```python
from build123d import *

# Parameters (mm, degrees)
SKETCH1_R           = 1.5
BOSS_EXTRUDE1_DEPTH = 25
SKETCH2_R           = 1.5
BOSS_EXTRUDE2_DEPTH = 2
SKETCH3_W           = 3
SKETCH3_H           = 17
CUT_EXTRUDE1_DEPTH  = 2
LPATTERN1_COUNT     = 7
LPATTERN1_PITCH     = 15


with BuildPart() as part:
    # Sketch1 → Boss-Extrude1 (new body)
    with BuildSketch(Plane.XY):
        with BuildLine():
            Line((-50.08587988, 100), (-70, 100))
            Line((-70, 100), (-70, -25.358547654))
            Line((-70, -25.358547654), (70, -25.358547654))
            Line((70, -25.358547654), (70, 30.840200363))
            ThreePointArc((70, 30.840200363), (67.647784394, 33.77119445), (66.543566366, 37.363456571))
            ThreePointArc((66.543566366, 37.363456571), (64.816659948, 40.011839547), (61.659897736, 40.187880739))
            ThreePointArc((61.659897736, 40.187880739), (57.09391383, 39.362702083), (52.647005809, 40.687140793))
            Line((52.647005809, 40.687140793), (21.252340591, 58.812859207))
            ThreePointArc((21.252340591, 58.812859207), (17.881889013, 62.001775167), (16.313522739, 66.368622551))
            ThreePointArc((16.313522739, 66.368622551), (14.584936491, 69.013139721), (11.430424316, 69.187880739))
            ThreePointArc((11.430424316, 69.187880739), (6.864440411, 68.362702083), (2.41753239, 69.687140793))
            Line((2.41753239, 69.687140793), (-28.977132828, 87.812859207))
            ThreePointArc((-28.977132828, 87.812859207), (-32.347584407, 91.001775167), (-33.915950681, 95.368622551))
            ThreePointArc((-33.915950681, 95.368622551), (-35.644536929, 98.013139721), (-38.799049103, 98.187880739))
            ThreePointArc((-38.799049103, 98.187880739), (-43.365033009, 97.362702083), (-47.81194103, 98.687140793))
            Line((-47.81194103, 98.687140793), (-50.08587988, 100))
        make_face()
        with BuildLine():
            Line((-50.621778265, 98), (68, 29.513684387))
            Line((68, 29.513684387), (68, -15.130655325))
            Line((68, -15.130655325), (51.241660417, -23.358547654))
            Line((51.241660417, -23.358547654), (-61.699771159, -23.358547654))
            Line((-61.699771159, -23.358547654), (-61.699771159, -19.718666382))
            ThreePointArc((-61.699771159, -19.718666382), (-63.017790644, -16.536685867), (-66.199771159, -15.218666382))
            Line((-66.199771159, -15.218666382), (-68, -15.218666382))
            Line((-68, -15.218666382), (-68, 98))
            Line((-68, 98), (-50.621778265, 98))
        make_face(mode=Mode.SUBTRACT)
        with Locations((63.06440991, 36.982050808)):
            Circle(SKETCH1_R, mode=Mode.SUBTRACT)
        with Locations((-37.394536929, 94.982050808)):
            Circle(SKETCH1_R, mode=Mode.SUBTRACT)
        with Locations((12.834936491, 65.982050808)):
            Circle(SKETCH1_R, mode=Mode.SUBTRACT)
        with Locations((65.552729719, -21.188668784)):
            Circle(SKETCH1_R, mode=Mode.SUBTRACT)
        with Locations((-66.199771159, -19.718666382)):
            Circle(SKETCH1_R, mode=Mode.SUBTRACT)
    extrude(amount=BOSS_EXTRUDE1_DEPTH)

    # Sketch2 → Boss-Extrude2 (add)
    with BuildSketch(Plane.XY.offset(25)):
        with BuildLine():
            Line((70, -25.358547654), (70, 30.840200363))
            ThreePointArc((70, 30.840200363), (67.647784394, 33.77119445), (66.543566366, 37.363456571))
            ThreePointArc((66.543566366, 37.363456571), (64.816659948, 40.011839547), (61.659897736, 40.187880739))
            ThreePointArc((61.659897736, 40.187880739), (57.09391383, 39.362702083), (52.647005809, 40.687140793))
            Line((52.647005809, 40.687140793), (21.252340591, 58.812859207))
            ThreePointArc((21.252340591, 58.812859207), (17.881889013, 62.001775167), (16.313522739, 66.368622551))
            ThreePointArc((16.313522739, 66.368622551), (14.584936491, 69.013139721), (11.430424316, 69.187880739))
            ThreePointArc((11.430424316, 69.187880739), (6.864440411, 68.362702083), (2.41753239, 69.687140793))
            Line((2.41753239, 69.687140793), (-28.977132828, 87.812859207))
            ThreePointArc((-28.977132828, 87.812859207), (-32.347584407, 91.001775167), (-33.915950681, 95.368622551))
            ThreePointArc((-33.915950681, 95.368622551), (-35.644536929, 98.013139721), (-38.799049103, 98.187880739))
            ThreePointArc((-38.799049103, 98.187880739), (-43.365033009, 97.362702083), (-47.81194103, 98.687140793))
            Line((-47.81194103, 98.687140793), (-50.08587988, 100))
            Line((-50.08587988, 100), (-70, 100))
            Line((-70, 100), (-70, -25.358547654))
            Line((-70, -25.358547654), (70, -25.358547654))
        make_face()
        with Locations((-37.394536929, 94.982050808)):
            Circle(SKETCH2_R, mode=Mode.SUBTRACT)
        with Locations((12.834936491, 65.982050808)):
            Circle(SKETCH2_R, mode=Mode.SUBTRACT)
        with Locations((63.06440991, 36.982050808)):
            Circle(SKETCH2_R, mode=Mode.SUBTRACT)
        with Locations((65.552729719, -21.188668784)):
            Circle(SKETCH2_R, mode=Mode.SUBTRACT)
        with Locations((-66.199771159, -19.718666382)):
            Circle(SKETCH2_R, mode=Mode.SUBTRACT)
    extrude(amount=BOSS_EXTRUDE2_DEPTH)

    # Sketch3 → Cut-Extrude1 (cut)
    with BuildSketch(Plane(origin=(0, -25.358547654, 0), x_dir=(-1, 0, 0), z_dir=(0, -1, 0))):
        with Locations((48.5, -13.5)):
            Rectangle(SKETCH3_W, SKETCH3_H)
    cut_extrude1 = extrude(amount=-CUT_EXTRUDE1_DEPTH, mode=Mode.SUBTRACT)

    # LPattern1: Cut-Extrude1 ×7
    with Locations(*[(i * LPATTERN1_PITCH, 0, 0) for i in range(1, LPATTERN1_COUNT)]):
        add(cut_extrude1, mode=Mode.SUBTRACT)


solid = part.part
```
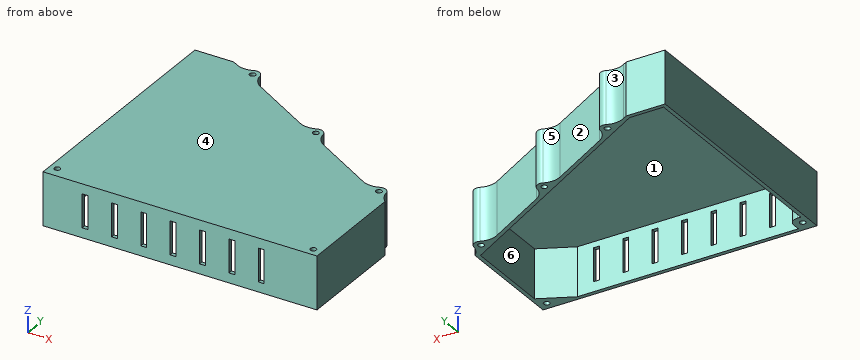
Work out the finished part from the listing and answer in its coordinate system (mm). Face numbers are marked on the shaded views. A direction names the side the tool comes from. Coordinates: 2 decimals unless noted, no trailing zeros. Loops run counter-clockwise (first coordinate to the right, second up) from the corner with the lowest first, then second, coordinate; pieces in that order, holes last. Notation, with made-up numbers: (-9, -20) -> (27, -20) arc R15 ccw to (27, -13) -> close; hole circle Ø8 at (51.5, 33). An arc over 180 degrees is marked (long way). Answer as CSV lines item,"result".
Q1. For a pull along X with two mould halves and no side action, classify the marked faces 1, 2, 3 and 4 as +X half, -X half, draft (parallel to the pull), parting line (faces both ways), or undercut.
Findings:
face 1,"undercut"
face 2,"+X half"
face 3,"undercut"
face 4,"draft"
Q2. A tool of negligible diameter and unlimited length cuts with its end or side. For the marked faces 5 and 6, from which of +Z, -Z, +X, -X, +Y, -Y can it reach the whole face along a straight path? Write none if from no direction.
Findings:
face 5,"+Z, -Z, +Y"
face 6,"-Z"
Q3. The part is cut by section C-C on z = 13. State how many separate pieces and enclosed holes the cut face has, and give its area (3 significant figures).
Findings:
separate pieces,"7"
enclosed holes,"5"
area,"1,130 mm²"
Q4. The part is cut by section B-B on y = 49. Write down the section's boundary in (x, z), and give its area (3 significant figures).
Findings:
outline,"(-70, 0) -> (-68, 0) -> (-68, 25) -> (34.25, 25) -> (34.25, 0) -> (38.25, 0) -> (38.25, 27) -> (-70, 27) -> close"
area,"366 mm²"
Q5. The part is cut by section A-A on x = -57.5. Write down the section's boundary in (y, z), and give its area (3 significant figures).
Findings:
outline,"(-25.36, 0) -> (-23.36, 0) -> (-23.36, 25) -> (98, 25) -> (98, 0) -> (100, 0) -> (100, 27) -> (-25.36, 27) -> close"
area,"351 mm²"
Q6. Find the intervals of material crossed by probe 1 along X at (y, z) = (-12.5, 20.25); probe 2 along X at (y, z) = (-19, 2); probe 3 along X at (y, z) = (-16, 18), in increasing order.
Findings:
probe 1,"x = -70 to -68, 68 to 70"
probe 2,"x = -70 to -67.52, -64.88 to -61.76, 60.12 to 70"
probe 3,"x = -70 to -63.67, 66.23 to 70"
Q7. Each of these flat-tipped pins is pushed along its axis until it touches: pin 1 (6 mm diameter, centred on x = 54, z = 16.5, fed in from +Y); pin 2 (1 mm diameter, centred on y = 35, z = 4, fed in from +X); pin 3 (12 mm diameter, centred on x = -41.5, z = 10, fed in from +Y). Where does it stop, or does it pass through?
Findings:
pin 1,"stops at y = 41.64"
pin 2,"stops at x = 67.3"
pin 3,"stops at y = 98.51"
